Here's how the part is built. I have some questions about the finished solid (model axes, mm). Face numbers are marked on the shaded views. A direction names the side the tool comes from. Coordinates: 2 decimals unless noted, no trailing zeros. Loops run counter-clockwise (first coordinate to the right, second up) from the corner with the lowest first, then second, coordinate; pieces in that order, holes last. Notation, with made-up numbers: M 1.5,38 L 60.5,38 A33 ccw 60.5,71 Z; hole C -30,11.25 d4. An arc over 180 degrees is marked long. Use one line per item in the form item = value. Start each with the question number.
(1) Will these pins go through, and if not, where does the flat tip stop? P1, Ø1, axis at x = 20, y = -49, coming from the +Z side; P2, Ø24, axis at x = 7, z = 1, coming from the -Y side; P3, Ø10, axis at x = -8, y = -15.5, coming from the +Z side.
(2) On a 3-axis mill with a long thin cutter (end or side, diameter ignored), from which of +Z, -Z, +X, -X, +Y, -Y can I reach the whole of each face in a straight line? I mean the marked faces 1, 2, 3, 4 and 5. Say none if no direction works.
(3) Imagine slicing it at B-B, the plane y = -47.5. Please give me the cut outline in (x, z), and give its area (3 significant figures).
(4) Imagine slicing it at C-C, the plane z = 21. Please give me the cut outline in (x, y), and give its area (3 significant figures).
(5) Imagine slicing it at A-A, the plane x = 0. Please give me the cut outline in (y, z), and give its area (3 significant figures).
(6) Imagine slicing it at D-D, the plane z = -1. Please give me the cut outline in (x, y), and give its area (3 significant figures).
(7) Please list where these lines run through material, in increasing order: L1, parallel to Z at x = 0, y = -7; L2, parallel to X at y = -4, z = 0; L3, parallel to X at y = -50, z = -28.
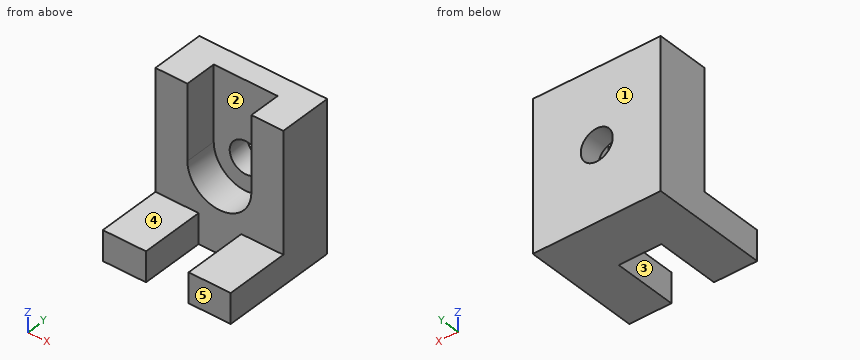
```python
from build123d import *

# Parameters (mm, degrees)
F0_W      = 60
F0_H      = 70
F1_DEPTH  = 25
F3_DEPTH  = 15
F4_R      = 7.5
F5_DEPTH  = 25
F5_FACE_R = 7.5
F6_DEPTH  = 25.001
F7_W      = 19.729286
F7_H      = 14
F7_W_2    = 20.270714
F8_DEPTH  = 30


with BuildPart() as f1:
    # F0 (on Front) → F1 (new body)
    with BuildSketch(Plane.XZ):
        Rectangle(F0_W, F0_H)
    extrude(amount=F1_DEPTH)

    # F2 (on face) → F3 (cut)
    with BuildSketch(Plane.XZ.offset(25)):
        with BuildLine():
            Line((-15, 35), (-15, 0))
            ThreePointArc((-15, 0), (0, -15), (15, 0))
            Line((15, 0), (15, 35))
            Line((15, 35), (-15, 35))
        make_face()
    extrude(amount=-F3_DEPTH, mode=Mode.SUBTRACT)

    # F4 (on Front) → F5 (join)
    with BuildSketch(Plane.XZ):
        Circle(F4_R)
    extrude(amount=F5_DEPTH)

    # F5_face (on face) → F6 (cut, through all)
    with BuildSketch(Plane.XZ.offset(25)):
        Circle(F5_FACE_R)
    extrude(amount=-F6_DEPTH, mode=Mode.SUBTRACT)

    # F7 (on face) → F8 (join)
    with BuildSketch(Plane.XZ.offset(25)):
        with Locations((20.135357, -28)):
            Rectangle(F7_W, F7_H)
        with Locations((-19.864643, -28)):
            Rectangle(F7_W_2, F7_H)
    extrude(amount=F8_DEPTH)


solid = f1.part
```
Answer:
q1.P1 = -21
q1.P2 = -25
q1.P3 = -7.48
q2.face_1 = +Z, -Z, +X, -X, +Y
q2.face_2 = +Z, -Y
q2.face_3 = +Z, -Z, -Y
q2.face_4 = +Z, +X, -X, -Y
q2.face_5 = +Z, -Z, +X, -X, -Y
q3.outline = M -30,-35 L -9.73,-35 L -9.73,-21 L -30,-21 Z; M 10.27,-35 L 30,-35 L 30,-21 L 10.27,-21 Z
q3.area = 560 mm²
q4.outline = M -30,-25 L -15,-25 L -15,-10 L 15,-10 L 15,-25 L 30,-25 L 30,0 L -30,0 Z
q4.area = 1,050 mm²
q5.outline = M -25,-35 L 0,-35 L 0,-7.5 L -10,-7.5 L -10,-15 L -25,-15 Z; M -10,7.5 L 0,7.5 L 0,35 L -10,35 Z
q5.area = 850 mm²
q6.outline = M -30,-25 L -14.97,-25 L -14.97,-10 L -7.43,-10 L -7.43,0 L -30,0 Z; M 7.43,-10 L 14.97,-10 L 14.97,-25 L 30,-25 L 30,0 L 7.43,0 Z
q6.area = 902 mm²
q7.L1 = -35 to -7.5, 7.5 to 35
q7.L2 = -30 to -7.5, 7.5 to 30
q7.L3 = -30 to -9.73, 10.27 to 30
